Build history of the part. All positions in model axes, mm. A direction names the side the tool comes from. Round coordinates to 2 decimals unless told otherwise and drop trailing zeros. Write each loop counter-clockwise with the first axis right and the second up, starting at its lowest first coordinate (ties: lowest second). Pieces come first, ordered by that corner, then holes.
Item 1: Band-saw the part on A-A, the plane y = 20. Count the separate pieces of the cut face and the enclosed holes in it, then the cut area to 3 significant figures.
Item 2: Drop flat-ended pins along their axis: pin 1 Ø0.5 at (y, z) = (10.5, 6.5) entering from -X; pin 2 Ø4.5 at (x, z) = (-13.5, 6.5) entering from +Y; pin 3 Ø1.5 at (x, z) = (37.5, 8) entering from +Y. Give the stop position or say it passes through.
Item 3: Band-saw the part on B-B, the plane x = 55. Write the cut outline in (y, z), then the cut area to 3 significant figures.
Item 4: 3-axis set-ups, long thin cutter, end or side, ignore diameter. For faces 1 (the flat face through (42.79, 14.04, 11.3)), 2 (the cylindrical face through (23.252, 5.357, 4.93)), 3 (the flat face through (50, 23, 8)): which of +Z, -Z, +X, -X, +Y, -Y reach the whole face in a straight line?
Item 5: Band-saw the part on D-D, the plane x = 28. Write the cut outline in (y, z).
Item 6: Wall check: probe 1 along X at (y, z) = (20.55, 7.5); probe 2 along Y at (x, z) = (20, 11.85); probe 3 along Y at (x, z) = (20, 2.75). Give the ranges that are in metal, low to high.
Item 7: Mould opens along X. For faces 4 (the flat face through (42, 29, 7)), 5 (the cylindrical face through (-17.745, 20.042, 2.139)), 6 (the cylindrical face through (55.751, 20.042, 9.885)) say: +X half, -X half, draft (parallel to the pull), parting line (faces both ways), or undercut.
Item 8: Band-saw the part on C-C, the plane z = 14. Write the cut outline in (x, y).
```python
from build123d import *

# Parameters (mm, degrees)
SKETCH1_W           = 40
SKETCH1_H           = 40
SKETCH1_R           = 6
BOSS_EXTRUDE1_DEPTH = 15
SKETCH2_R           = 15
CUT_EXTRUDE1_DEPTH  = 10
SKETCH4_R           = 4
BOSS_EXTRUDE2_DEPTH = 15
SKETCH5_R           = 5
BOSS_EXTRUDE3_DEPTH = 5
BOSS_EXTRUDE4_START = 5
SKETCH7_R           = 5
BOSS_EXTRUDE4_DEPTH = 5
BOSS_EXTRUDE5_START = 10
SKETCH8_R           = 4
BOSS_EXTRUDE5_DEPTH = 10
FILLET1_R           = 10
SKETCH9_W           = 15
SKETCH9_H           = 6
BOSS_EXTRUDE6_DEPTH = 20
SKETCH10_W          = 15
SKETCH10_H          = 6
BOSS_EXTRUDE7_DEPTH = 20
CUT_EXTRUDE2_REACH  = 74.588
SKETCH11_R          = 2.5
FILLET2_R           = 7.5
BOSS_EXTRUDE8_DEPTH = 6
BOSS_EXTRUDE9_DEPTH = 6


with BuildPart() as part:
    # Sketch1 → Boss-Extrude1 (new body)
    with BuildSketch(Plane.XY):
        with Locations((20, 20)):
            Rectangle(SKETCH1_W, SKETCH1_H)
        with Locations((20, 20)):
            Circle(SKETCH1_R, mode=Mode.SUBTRACT)
    extrude(amount=BOSS_EXTRUDE1_DEPTH)

    # Sketch2 → Cut-Extrude1 (cut)
    with BuildSketch(Plane(origin=(0, 0, 0), x_dir=(-1, 0, 0), z_dir=(0, 0, -1))):
        with Locations((-20, 20)):
            Circle(SKETCH2_R)
    extrude(amount=-CUT_EXTRUDE1_DEPTH, mode=Mode.SUBTRACT)

    # Sketch4 → Boss-Extrude2 (add)
    with BuildSketch(Plane(origin=(0, 40, 0), x_dir=(1, 0, 0), z_dir=(0, 1, 0))):
        with Locations((20, -5)):
            Circle(SKETCH4_R)
    extrude(amount=BOSS_EXTRUDE2_DEPTH)

    # Sketch5 → Boss-Extrude3 (add)
    with BuildSketch(Plane(origin=(0, 40, 0), x_dir=(1, 0, 0), z_dir=(0, 1, 0))):
        with Locations(Location((20, -5, 0), (0, 0, 90))):
            Circle(SKETCH5_R)
    extrude(amount=BOSS_EXTRUDE3_DEPTH)

    # Sketch7 → Boss-Extrude4 (add)
    with BuildSketch(Plane.XZ.offset(BOSS_EXTRUDE4_START)):
        with Locations(Location((20, 5, 0), (0, 0, 270))):
            Circle(SKETCH7_R)
    extrude(amount=-BOSS_EXTRUDE4_DEPTH)

    # Sketch8 → Boss-Extrude5 (add)
    with BuildSketch(Plane.XZ.offset(5).offset(BOSS_EXTRUDE5_START)):
        with Locations(Location((20, 5, 0), (0, 0, 180))):
            Circle(SKETCH8_R)
    extrude(amount=-BOSS_EXTRUDE5_DEPTH)

    # Fillet1
    fillet1_edges = [part.edges().sort_by_distance(p)[0] for p in [
        (40, 0, 7.5),
        (0, 0, 7.5),
        (0, 40, 7.5),
        (40, 40, 7.5),
    ]]
    fillet(fillet1_edges, radius=FILLET1_R)

    # Sketch9 → Boss-Extrude6 (add)
    with BuildSketch(Plane(origin=(40, 0, 0), x_dir=(0, 0, -1), z_dir=(1, 0, 0))):
        with Locations((-7.5, 20)):
            Rectangle(SKETCH9_W, SKETCH9_H)
    extrude(amount=BOSS_EXTRUDE6_DEPTH)

    # Sketch10 → Boss-Extrude7 (add)
    with BuildSketch(Plane.ZY):
        with Locations((7.5, 20)):
            Rectangle(SKETCH10_W, SKETCH10_H)
    extrude(amount=BOSS_EXTRUDE7_DEPTH)

    # Sketch11 → Cut-Extrude2 (cut, up to next)
    with BuildSketch(Plane(origin=(0, 23, 0), x_dir=(1, 0, 0), z_dir=(0, 1, 0)), mode=Mode.PRIVATE) as cut_extrude2_sk1:
        with Locations(Location((-15, -7.5, 0), (0, 0, 270))):
            Circle(SKETCH11_R)
    cut_extrude2_tool1 = extrude(cut_extrude2_sk1.sketch, amount=-CUT_EXTRUDE2_REACH, mode=Mode.PRIVATE) & part.part
    # Sketch11 → Cut-Extrude2 (cut, up to next)
    with BuildSketch(Plane(origin=(0, 23, 0), x_dir=(1, 0, 0), z_dir=(0, 1, 0)), mode=Mode.PRIVATE) as cut_extrude2_sk2:
        with Locations(Location((55, -7.5, 0), (0, 0, 270))):
            Circle(SKETCH11_R)
    cut_extrude2_tool2 = extrude(cut_extrude2_sk2.sketch, amount=-CUT_EXTRUDE2_REACH, mode=Mode.PRIVATE) & part.part
    add(cut_extrude2_tool1.solids().sort_by_distance((-15, 23, 7.5))[0], mode=Mode.SUBTRACT)
    add(cut_extrude2_tool2.solids().sort_by_distance((55, 23, 7.5))[0], mode=Mode.SUBTRACT)

    # Fillet2
    fillet2_edges = [part.edges().sort_by_distance(p)[0] for p in [
        (-20, 20, 15),
        (-20, 20, 0),
        (60, 20, 15),
        (60, 20, 0),
    ]]
    fillet(fillet2_edges, radius=FILLET2_R - 0.0001)  # a hair under: the kernel refuses the full size

    # Sketch12 → Boss-Extrude8 (add)
    with BuildSketch(Plane(origin=(0, 23, 0), x_dir=(1, 0, 0), z_dir=(0, 1, 0))):
        Polygon((0, 0), (0, -15), (-5.651655376, -7.5), align=None)
        Polygon((45.651655376, -7.5), (40, -15), (40, 0), align=None)
    extrude(amount=BOSS_EXTRUDE8_DEPTH)

    # Sketch13 → Boss-Extrude9 (add)
    with BuildSketch(Plane.XZ.offset(-17)):
        Polygon((0, 15), (-5.651655376, 7.5), (0, 0), align=None)
        Polygon((40, 15), (45.651655376, 7.5), (40, 0), align=None)
    extrude(amount=BOSS_EXTRUDE9_DEPTH)


solid = part.part
```
Results:
1. separate pieces: 2
1. enclosed holes: 2
1. area: 752 mm2
2. pin 1: stops at x = 0
2. pin 2: stops at y = 23
2. pin 3: stops at y = 37.38
3. outline: (17, 0.43) - (23, 0.43) - (23, 5) - (17, 5) - close; (17, 10) - (23, 10) - (23, 14.57) - (17, 14.57) - close
3. area: 54.9 mm2
4. face 1: +Z, +X, -Y
4. face 2: -Z
4. face 3: +X, +Y
5. outline: (0, 0) - (7.31, 0) - (7.31, 10) - (32.69, 10) - (32.69, 0) - (40, 0) - (40, 15) - (0, 15) - close
6. probe 1: x = -20 to -17.5, -12.5 to 5.01, 34.99 to 52.5, 57.5 to 60
6. probe 2: y = 0 to 14, 26 to 40
6. probe 3: y = -15 to 5, 35 to 55
7. face 4: draft
7. face 5: -X half
7. face 6: undercut
8. outline: (-16.24, 17) - (-0.75, 17) - (-0.75, 11) - (0, 11) - (0, 10) arc R10 ccw to (10, 0) - (30, 0) arc R10 ccw to (40, 10) - (40, 11) - (40.75, 11) - (40.75, 17) - (56.24, 17) - (56.24, 23) - (40.75, 23) - (40.75, 29) - (40, 29) - (40, 30) arc R10 ccw to (30, 40) - (10, 40) arc R10 ccw to (0, 30) - (0, 29) - (-0.75, 29) - (-0.75, 23) - (-16.24, 23) - close; hole circle Ø12 at (20, 20)
